from build123d import *

# Parameters (mm, degrees)
F3_R     = 25.4
F4_R     = 4.7625
F5_DEPTH = 9.525
F6_R     = 1.5875
F7_DEPTH = 9.525


# Not quite as in the source:
# - a fillet or chamfer that OpenCascade refuses, or shapes differently, is made with other operations: its cross-section is extruded or revolved along the edge and cut away or added


with BuildPart() as f1:
    # F0 (on Front) → F1 (revolve)
    with BuildSketch(Plane.XZ):
        Polygon((10.5000606809, 4.0159458295), (31.75, 8.134865202), (31.75, 28.454865202), (24.4433090497, 28.454865202), (7.62, 9.4384327507), (7.62, 45.72), (0, 45.72), (0, 0), (1.5875, 0), align=None)
    revolve(axis=Axis((0, 0, 22.86), (0, 0, -1)))

    # F2: fillet of radius 10.16 on 3 edges, made by hand

    # F2_s1 → F2_t2 (revolve, cut)
    with BuildSketch(Plane.XZ):
        with BuildLine():
            ThreePointArc((23.5233497224, 6.5402766862), (29.4279982514, 10.0500062027), (31.75, 16.5146317456))
            Line((31.75, 16.5146317456), (31.75, 8.134865202))
            Line((31.75, 8.134865202), (23.5233497224, 6.5402766862))
        make_face()
    revolve(axis=Axis((0, 0, 8.134865202), (0, 0, -1)), mode=Mode.SUBTRACT)

    # F2_s3 → F2_t4 (revolve, cut)
    with BuildSketch(Plane.XZ):
        with BuildLine():
            ThreePointArc((31.75, 18.7037510366), (29.7206586432, 24.7962045676), (24.4433090497, 28.454865202))
            Line((24.4433090497, 28.454865202), (31.75, 28.454865202))
            Line((31.75, 28.454865202), (31.75, 18.7037510366))
        make_face()
    revolve(axis=Axis((0, 0, 28.454865202), (0, 0, -1)), mode=Mode.SUBTRACT)

    # F3
    f3_edges = [f1.edges().sort_by_distance(p)[0] for p in [
        (-10.500061, 0, 4.015946),
    ]]
    fillet(f3_edges, radius=F3_R)

    # F4 (on face) → F5 (cut)
    with BuildSketch(Plane.XY.offset(45.72)):
        Circle(F4_R)
    extrude(amount=-F5_DEPTH, mode=Mode.SUBTRACT)

    # F6 (on Top) → F7 (cut)
    with BuildSketch(Plane.XY):
        Circle(F6_R)
    extrude(amount=F7_DEPTH, mode=Mode.SUBTRACT)


solid = f1.part
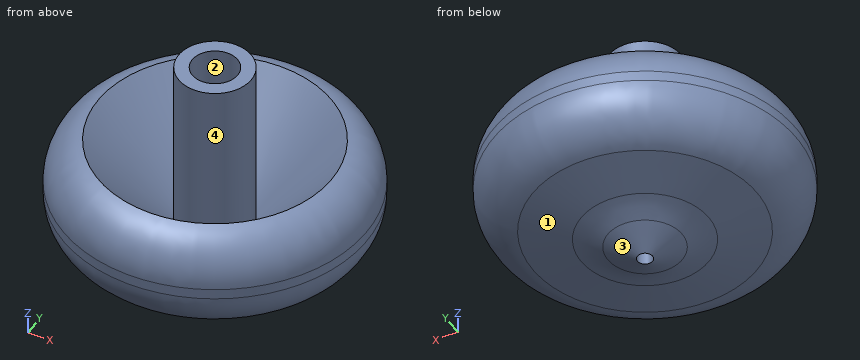
The listing builds one solid part. Answer for the finished solid, in the listing's coordinates (mm). Face numbers are marked on the shaded views. A direction names the side the tool comes from. Coordinates: 2 decimals unless noted, no trailing zeros. Loops run counter-clockwise (first coordinate to the right, second up) from the corner with the lowest first, then second, coordinate; pieces in that order, holes last.
1) Find the intervals of material crossed by L1, parallel to Y at x = 0, z = 41; L2, parallel to Y at x = -3, z = 23; L3, parallel to X at y = -6, z = 21, in increasing order.
2) Flat-ended cylindrical pins translate along their axes: pin 1 Ø11 at (x, y) = (0, 0) entering from -Z; pin 2 Ø4 at (y, z) = (-3.5, 11.5) entering from +X; pin 3 Ø5 at (x, y) = (-19.5, 20) entering from +Z; pin 4 Ø6 at (y, z) = (-16, 20.5) entering from +X. Find the tip coordinate at first contact, or state that the pin passes through.
3) Find section A-A on z = 20. Write down the section's boundary in (x, y), then the cut area to 3 significant figures.
4) A tool of negligible diameter and unlimited length cuts with its end or side. For the marked faces 1 and 2, from which of +Z, -Z, +X, -X, +Y, -Y can it reach the whole face along a straight path? Write none if from no direction.
5) Find section B-B on z = 34. Write down the section's boundary in (x, y).
6) Determine the mould class of the marked faces 3 and 4 for opening direction Y: pulls with the +Y half, pulls with the -Y half, needs draft (parallel to the pull), parting line crosses it, or undercut.
Values:
1. L1: y = -7.62 to -4.76, 4.76 to 7.62
1. L2: y = -30.65 to -19.39, -7 to 7, 19.39 to 30.65
1. L3: x = -30.91 to -16.81, -4.7 to 4.7, 16.81 to 30.91
2. pin 1: stops at z = 0
2. pin 2: stops at x = 31.13
2. pin 3: stops at z = 28.11
2. pin 4: stops at x = 28.86
3. outline: circle Ø63.33 at (0, 0); circle Ø15.24 at (0, 0); hole circle Ø33.93 at (0, 0)
3. area: 2,430 mm2
4. face 1: -Z
4. face 2: +Z
5. outline: circle Ø15.24 at (0, 0)
6. face 3: parting line crosses it
6. face 4: undercut
